from build123d import *

# Parameters (mm, degrees)
F0_W     = 35.2
F0_H     = 35.200004
F0_R     = 1.767695
F0_R_2   = 11
F0_R_3   = 2.5
F1_DEPTH = 37
F2_DEPTH = 2
F3_DEPTH = 21
F4_SIZE  = 3


with BuildPart() as f1:
    # F0 (on Front) → F1 (new body)
    with BuildSketch(Plane.XZ):
        Rectangle(F0_W, F0_H)
        with Locations((-13, -14.419172)):
            Circle(F0_R, mode=Mode.SUBTRACT)
        with Locations((13, -14.419172)):
            Circle(F0_R, mode=Mode.SUBTRACT)
        with Locations((-13, 14.419172)):
            Circle(F0_R, mode=Mode.SUBTRACT)
        Circle(F0_R_2, mode=Mode.SUBTRACT)
        with Locations((13, 14.419172)):
            Circle(F0_R, mode=Mode.SUBTRACT)
        Circle(F0_R_2)
        Circle(F0_R_3, mode=Mode.SUBTRACT)
        Circle(F0_R_3)
    extrude(amount=-F1_DEPTH)

    # F0 (on Front) → F2 (join)
    with BuildSketch(Plane.XZ):
        Circle(F0_R_2)
        Circle(F0_R_3, mode=Mode.SUBTRACT)
    extrude(amount=F2_DEPTH)

    # F0 (on Front) → F3 (join)
    with BuildSketch(Plane.XZ):
        Circle(F0_R_3)
    extrude(amount=F3_DEPTH)

    # F4
    f4_edges = [f1.edges().sort_by_distance(p)[0] for p in [
        (17.6, 18.5, 17.600002),
        (-17.6, 18.5, 17.600002),
        (17.6, 18.5, -17.600002),
        (-17.6, 18.5, -17.600002),
    ]]
    chamfer(f4_edges, length=F4_SIZE)


solid = f1.part
Build history of the part. All positions in model axes, mm. A direction names the side the tool comes from. Coordinates: 2 decimals unless noted, no trailing zeros. Order: outer loops, then holes, each group sorted by start corner. A loop starts at its lowest first (then second) coordinate and runs counter-clockwise, first axis right, second up. Notation, with made-up numbers: (33, 3) -> (53, 3) arc R21 cw to (53, 21) -> close; hole circle Ø5 at (-36.75, 77.25). An arc over 180 degrees is marked (long way). One line per item, written item: value.
(1) Tool access for faces 4 (the cylindrical face through (-2.38, -0.99, -10.74)), 5 (the flat face through (0, -21, 0)): list every direction of +Z, -Z, +X, -X, +Y, -Y with a clear straight run to the whole face (end or side of a thin tool).
Checked values:
face 4: -Y
face 5: +Z, -Z, +X, -X, -Y
(2) Drop flat-ended pins along their axis: pin 1 Ø2 at (x, z) = (-13, 14.42) entering from -Y; pin 2 Ø1 at (y, z) = (-13, -1.5) entering from +X; pin 3 Ø6 at (x, z) = (7.5, -5.5) entering from -Y. Give the stop position or say it passes through.
Checked values:
pin 1: through
pin 2: x = 2.29
pin 3: y = -2
(3) Slice it at D-D, the plane x = 0. List the corners of the cut face in (y, z), plus the area to 3 significant figures.
Checked values:
outline: (-21, -2.5) -> (-2, -2.5) -> (-2, -11) -> (0, -11) -> (0, -17.6) -> (37, -17.6) -> (37, 17.6) -> (0, 17.6) -> (0, 11) -> (-2, 11) -> (-2, 2.5) -> (-21, 2.5) -> close
area: 1,440 mm2
(4) Slice it at B-B, the plane z = 0. List the corners of the cut face in (x, y), plus the area to 3 significant figures.
Checked values:
outline: (-17.6, 0) -> (-11, 0) -> (-11, -2) -> (-2.5, -2) -> (-2.5, -21) -> (2.5, -21) -> (2.5, -2) -> (11, -2) -> (11, 0) -> (17.6, 0) -> (17.6, 37) -> (-17.6, 37) -> close
area: 1,440 mm2
(5) Slice it at A-A, the plane x = 13. List the corners of the cut face in (y, z).
Checked values:
outline: (0, -17.6) -> (37, -17.6) -> (37, -16.19) -> (0, -16.19) -> close; (0, -12.65) -> (37, -12.65) -> (37, 12.65) -> (0, 12.65) -> close; (0, 16.19) -> (37, 16.19) -> (37, 17.6) -> (0, 17.6) -> close
(6) Slice it at C-C, the plane y = 7. List the corners of the cut face in (x, z).
Checked values:
outline: (-17.6, -14.6) -> (-14.6, -17.6) -> (14.6, -17.6) -> (17.6, -14.6) -> (17.6, 14.6) -> (14.6, 17.6) -> (-14.6, 17.6) -> (-17.6, 14.6) -> close; hole circle Ø3.54 at (-13, -14.42); hole circle Ø3.54 at (-13, 14.42); hole circle Ø3.54 at (13, -14.42); hole circle Ø3.54 at (13, 14.42)
(7) Probe line 1 (Z direction, x = 13, y = 19); line 2 (X direction, y = 11.5, z = -15); line 3 (Z direction, x = -12, y = 27.5). List the from-to ranges inside material, lowest first. Write a range as [from, to].
Checked values:
line 1: [-17.6, -16.19], [-12.65, 12.65], [16.19, 17.6]
line 2: [-17.2, -14.67], [-11.33, 11.33], [14.67, 17.2]
line 3: [-17.6, -15.88], [-12.96, 12.96], [15.88, 17.6]
(8) Mould opens along X. For faces 1 (the cylindrical face through (-0.54, -11.37, -2.44)), 2 (the cylindrical face through (-12.05, 18.24, -12.93)), 3 (the flat face through (0, 37, 0)) say: pulls with the +X half, pulls with the -X half, needs draft (parallel to the pull), parting line crosses it, or undercut.
Checked values:
face 1: parting line crosses it
face 2: undercut
face 3: needs draft
